from build123d import *

# Parameters (mm, degrees)
BOSS_EXTRUDE1_DEPTH = 19.5


with BuildPart() as part:
    # Sketch1 → Boss-Extrude1 (new body)
    with BuildSketch(Plane(origin=(0, 0, 0), x_dir=(0, 1, 0), z_dir=(0, 0, 1))):
        with BuildLine():
            Line((8.15, 18.15), (8.15, 20.15))
            ThreePointArc((8.15, 20.15), (7.271320344, 22.271320344), (5.15, 23.15))
            Line((5.15, 23.15), (1.15, 23.15))
            Line((1.15, 23.15), (1.15, 20.15))
            Line((1.15, 20.15), (3.15, 20.15))
            ThreePointArc((3.15, 20.15), (4.564213562, 19.564213562), (5.15, 18.15))
            Line((5.15, 18.15), (5.15, -18.15))
            ThreePointArc((5.15, -18.15), (4.564213562, -19.564213562), (3.15, -20.15))
            Line((3.15, -20.15), (-33.15, -20.15))
            ThreePointArc((-33.15, -20.15), (-34.564213562, -19.564213562), (-35.15, -18.15))
            Line((-35.15, -18.15), (-35.15, 18.15))
            ThreePointArc((-35.15, 18.15), (-34.564213562, 19.564213562), (-33.15, 20.15))
            Line((-33.15, 20.15), (-31.15, 20.15))
            Line((-31.15, 20.15), (-31.15, 23.15))
            Line((-31.15, 23.15), (-35.15, 23.15))
            ThreePointArc((-35.15, 23.15), (-37.271320344, 22.271320344), (-38.15, 20.15))
            Line((-38.15, 20.15), (-38.15, -20.15))
            ThreePointArc((-38.15, -20.15), (-37.271320344, -22.271320344), (-35.15, -23.15))
            Line((-35.15, -23.15), (5.15, -23.15))
            ThreePointArc((5.15, -23.15), (7.271320344, -22.271320344), (8.15, -20.15))
            Line((8.15, -20.15), (8.15, 18.15))
        make_face()
    extrude(amount=BOSS_EXTRUDE1_DEPTH)


solid = part.part
Geometry check sheet. Reference: the model listing, model coordinates, mm. A direction names the side the tool comes from. Round coordinates to 2 decimals unless told otherwise and drop trailing zeros. Loops run counter-clockwise (first coordinate to the right, second up) from the corner with the lowest first, then second, coordinate; pieces in that order, holes last. Notation, with made-up numbers: (65, -36) -> (114, -36) arc R26 ccw to (114, -4) -> close; hole circle Ø6 at (40.25, 30). An arc over 180 degrees is marked (long way). Answer as a JSON object with one key per item and string values. Group by question number.
Item 1: Release check for a two-part mould opening along Y. For faces 1 (the face through (20.5, -15.1, 19.5)), 2 (the face through (-20.15, -32, 10)), 3 (the face through (-22.29, -37.25, 9.61)) record: pulls with the +Y half, pulls with the -Y half, needs draft (parallel to the pull), parting line crosses it, or undercut.
Item 2: Depth check by flat-ended pin: pin 1 Ø1.5 at (x, z) = (-22, 13) entering from -Y; pin 2 Ø2.5 at (x, z) = (-21, 12) entering from +Y. Enter the tip coordinate at first touch or a pass-through.
Item 3: Cross-section at A-A, the plane x = -8. Record the cut outline in (y, z).
Item 4: Cross-section at D-D, the plane y = -3. Record the cut outline in (x, z).
Item 5: Thickness scan on line 1 along X through (y, z) = (2.5, 2.25); line 2 along Y through (x, z) = (-2, 18.75); line 3 along X through (y, z) = (-17.5, 14.75). Record the ranges inside material, lowest first.
Item 6: Cross-section at B-B, the plane z = 15.25. Record the cut outline in (x, y), plus the area to 3 significant figures.
Item 7: Cross-section at C-C, the plane x = -19. Record the cut outline in (y, z).
Item 8: Set-up check for faces 4 (the face through (-22, 1.15, 10)), 5 (the face through (0, 5.15, 10)), 6 (the face through (23.15, -15, 10)): record each of +Z, -Z, +X, -X, +Y, -Y from which the full face is reachable in a straight line by a thin tool's end or side.
Determined:
{
 "1": {"face 1": "needs draft", "face 2": "undercut", "face 3": "pulls with the -Y half"},
 "2": {"pin 1": "stops at y = -37.94", "pin 2": "stops at y = 8.15"},
 "3": {"outline": "(-38.15, 0) -> (-35.15, 0) -> (-35.15, 19.5) -> (-38.15, 19.5) -> close; (5.15, 0) -> (8.15, 0) -> (8.15, 19.5) -> (5.15, 19.5) -> close"},
 "4": {"outline": "(20.15, 0) -> (23.15, 0) -> (23.15, 19.5) -> (20.15, 19.5) -> close"},
 "5": {"line 1": "x = -23.15 to -20.15, 20.15 to 23.15", "line 2": "y = -38.15 to -35.15, 5.15 to 8.15", "line 3": "x = 20.15 to 23.15"},
 "6": {"outline": "(-23.15, -35.15) arc R3 ccw to (-20.15, -38.15) -> (20.15, -38.15) arc R3 ccw to (23.15, -35.15) -> (23.15, 5.15) arc R3 ccw to (20.15, 8.15) -> (-20.15, 8.15) arc R3 ccw to (-23.15, 5.15) -> (-23.15, 1.15) -> (-20.15, 1.15) -> (-20.15, 3.15) arc R2 cw to (-18.15, 5.15) -> (18.15, 5.15) arc R2 cw to (20.15, 3.15) -> (20.15, -33.15) arc R2 cw to (18.15, -35.15) -> (-18.15, -35.15) arc R2 cw to (-20.15, -33.15) -> (-20.15, -31.15) -> (-23.15, -31.15) -> close", "area": "418 mm²"},
 "7": {"outline": "(-38.15, 0) -> (-34.96, 0) -> (-34.96, 19.5) -> (-38.15, 19.5) -> close; (4.96, 0) -> (8.15, 0) -> (8.15, 19.5) -> (4.96, 19.5) -> close"},
 "8": {"face 4": "+Z, -Z, -X", "face 5": "+Z, -Z", "face 6": "+Z, -Z, +X, +Y, -Y"}
}
